Can you work these out from the drawing? Everything is in mm from the part's minimum corner. Round coordinates to 2 decimals unless told otherwise and drop trailing zeros. Order: outer loops, then holes, each group sorted by start corner. A loop starts at its lowest first (then second) coordinate and runs counter-clockwise, first axis right, second up. Notation, with made-up numbers: (33.25, -29.5) - (67.25, -29.5) arc R16 cw to (67.25, 0.5) - close; hole circle Ø8 at (-4, -15.75). An arc over 180 degrees is marked (long way). Answer as a JSON object with one key per item and string values.
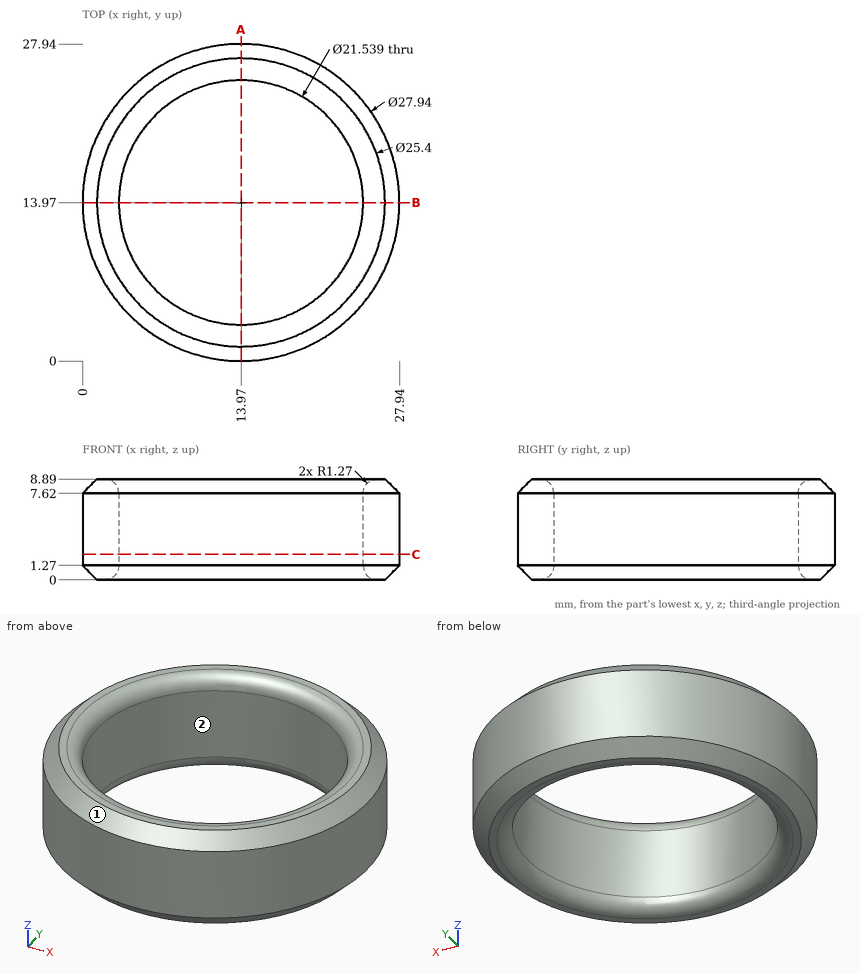
1. Thinking about a two-plate mould opening in Y: for the marked faces 1 and 2, which applies, pulls with the +Y half, pulls with the -Y half, needs draft (parallel to the pull), parting line crosses it, or undercut?
Responses:
{"face 1": "parting line crosses it", "face 2": "undercut"}
2. For P1, Ø3, axis at x = 3.5, z = 5.5, coming from the -Y side; P2, Ø5, axis at y = 18.5, z = 4, coming from the -X side; P3, Ø5, axis at y = 7, z = 1.5, coming from the -X side; P4, Ø5, axis at y = 12, z = 3.5, coming from the -X side, each with a flat end and sliding along its axis, tell me the tip position at first contact or that it passes through.
Responses:
{"P1": "y = 3.26", "P2": "x = 0.15", "P3": "x = 0.73", "P4": "x = 0"}
3. Imagine slicing it at C-C (z = 2.25). List the corners of the cut face in (x, y) for me.
Responses:
{"outline": "circle Ø27.94 at (13.97, 13.97); hole circle Ø21.54 at (13.97, 13.97)"}
4. Imagine slicing it at A-A (x = 13.97). List the corners of the cut face in (y, z) for me, plus the area to 3 significant figures.
Responses:
{"outline": "(0, 1.27) - (1.27, 0) - (1.93, 0) arc R1.27 ccw to (3.2, 1.27) - (3.2, 7.62) arc R1.27 ccw to (1.93, 8.89) - (1.27, 8.89) - (0, 7.62) - close; (24.74, 1.27) arc R1.27 ccw to (26.01, 0) - (26.67, 0) - (27.94, 1.27) - (27.94, 7.62) - (26.67, 8.89) - (26.01, 8.89) arc R1.27 ccw to (24.74, 7.62) - close", "area": "52.3 mm2"}
5. If I drill on L1, parallel to Y at x = 13.97, z = 5.75; L2, parallel to X at y = 4.75, z = 4.75 (1 decimal); L3, parallel to X at y = 4, z = 8 (1 decimal), over which ranges is the centre line in solid material (lowest first)? Write a range as [from, to].
Responses:
{"L1": "[0, 3.2], [24.74, 27.94]", "L2": "[3.5, 8.4], [19.5, 24.5]", "L3": "[4.7, 9.7], [18.2, 23.2]"}
